```python
from build123d import *

# Parameters (mm, degrees)
SKETCH_1_W          = 38.4
SKETCH_1_H          = 30
EXTRUDE_1_DEPTH     = 2
CUT_EXTRUDE_1_DEPTH = 2
SKETCH_3_W          = 23
SKETCH_3_H          = 6
EXTRUDE_2_DEPTH     = 2
SKETCH_4_R          = 1.05
CUT_EXTRUDE_2_DEPTH = 2
SKETCH_5_W          = 7
SKETCH_5_H          = 3
EXTRUDE_3_DEPTH     = 2


with BuildPart() as part:
    # 草图1 → 凸台-拉伸1 (new body)
    with BuildSketch(Plane.XY):
        Rectangle(SKETCH_1_W, SKETCH_1_H)
    extrude(amount=EXTRUDE_1_DEPTH)

    # 草图2 → 切除-拉伸1 (cut)
    with BuildSketch(Plane(origin=(0, 0, 0), x_dir=(-1, 0, 0), z_dir=(0, 0, -1))):
        with BuildLine():
            Line((-12.2, 1.5), (-12.2, 15))
            Line((-12.2, 15), (12.2, 15))
            Line((12.2, 15), (12.2, 1.5))
            ThreePointArc((12.2, 1.5), (0, -10.7), (-12.2, 1.5))
        make_face()
    extrude(amount=-CUT_EXTRUDE_1_DEPTH, mode=Mode.SUBTRACT)

    # 草图3 → 凸台-拉伸2 (add)
    with BuildSketch(Plane(origin=(0, 0, 0), x_dir=(-1, 0, 0), z_dir=(0, 0, -1))):
        with Locations((0, -15)):
            Rectangle(SKETCH_3_W, SKETCH_3_H)
    extrude(amount=-EXTRUDE_2_DEPTH)

    # 草图4 → 切除-拉伸2 (cut)
    with BuildSketch(Plane.XY.offset(2)):
        with Locations((12.55, -15)):
            Circle(SKETCH_4_R)
        with Locations((-12.55, -15)):
            Circle(SKETCH_4_R)
    extrude(amount=-CUT_EXTRUDE_2_DEPTH, mode=Mode.SUBTRACT)

    # 草图5 → 凸台-拉伸3 (add)
    with BuildSketch(Plane(origin=(0, 0, 0), x_dir=(-1, 0, 0), z_dir=(0, 0, -1))):
        with Locations((-15.7, 16.5)):
            Rectangle(SKETCH_5_W, SKETCH_5_H)
        with Locations((15.7, 16.5)):
            Rectangle(SKETCH_5_W, SKETCH_5_H)
    extrude(amount=-EXTRUDE_3_DEPTH)


solid = part.part
```
For this review, take the finished solid that the model builds, in its own axes (mm). A direction names the side the tool comes from. Coordinates: 2 decimals unless noted, no trailing zeros. Write each loop counter-clockwise with the first axis right and the second up, starting at its lowest first coordinate (ties: lowest second). Pieces come first, ordered by that corner, then holes. Notation, with made-up numbers: (84, 20) - (100, 20) arc R24 cw to (100, 52) - close; hole circle Ø1 at (-19.75, 41.5). An arc over 180 degrees is marked (long way). Answer in a Markdown table with one row per item. Add a question column.
Q1. We need section B-B, the plane z = 0.6. State the section outline as (x, y) points.
Q2. We need section A-A, the plane y = 15.5. State the section outline as (x, z) points.
Q3. Tool access review of faces 1 (the flat face through (11.5, -17, 1)), 2 (the flat face through (-16, -15, 1)), 3 (the flat face through (12.2, 10, 1)): name each direction out of +Z, -Z, +X, -X, +Y, -Y from which nothing blocks a thin tool from reaching the whole face with its end or side.
Q4. We need section C-C, the plane y = -2.5. State the section outline as (x, z) points, and give its area (3 significant figures).
Q5. For P1, Ø1, axis at x = 15.5, z = 0.5, coming from the -Y side; P2, Ø0.6, axis at y = -16, z = 1, coming from the -X side, all flat-tipped, find the tip position at first contact; note any pin that passes through.
Q6. Draft analysis for pull direction X (two halves, no side actions). For faces 4 (the flat face through (0, -12, 0)), 5 (the flat face through (-19.2, 1, 1)), 6 (the cylindrical face through (12.57, -13.95, 1.01)), state which applies: +X half, -X half, draft (parallel to the pull), parting line (faces both ways), or undercut.
Q7. For probe 1 along X at (y, z) = (7, 0.7); probe 2 along X at (y, z) = (-4.5, 0.5); probe 3 along Y at (x, z) = (-16.5, 0.1), list the stretches that pass through material, from the lowest coordinate up.
Q8. We need section D-D, the plane x = 0. State the section outline as (y, z) points, and give its area (3 significant figures).
Answer list:
| question | item | result |
|---|---|---|
| 1 | outline | (-19.2, -15) - (-13.6, -15) arc R1.05 cw to (-11.5, -15) - (-11.5, -18) - (11.5, -18) - (11.5, -15) arc R1.05 cw to (13.6, -15) - (19.2, -15) - (19.2, 18) - (12.2, 18) - (12.2, 1.5) arc R12.2 cw to (-12.2, 1.5) - (-12.2, 18) - (-19.2, 18) - close |
| 2 | outline | (-19.2, 0) - (-12.2, 0) - (-12.2, 2) - (-19.2, 2) - close; (12.2, 0) - (19.2, 0) - (19.2, 2) - (12.2, 2) - close |
| 3 | face 1 | +Z, -Z, +X, -Y |
| 3 | face 2 | +Z, -Z, -X, -Y |
| 3 | face 3 | +Z, -Z, +Y |
| 4 | outline | (-19.2, 0) - (-11.53, 0) - (-11.53, 2) - (-19.2, 2) - close; (11.53, 0) - (19.2, 0) - (19.2, 2) - (11.53, 2) - close |
| 4 | area | 30.7 mm2 |
| 5 | P1 | stops at y = -15 |
| 5 | P2 | stops at x = -11.5 |
| 6 | face 4 | draft |
| 6 | face 5 | -X half |
| 6 | face 6 | undercut |
| 7 | probe 1 | x = -19.2 to -12.2, 12.2 to 19.2 |
| 7 | probe 2 | x = -19.2 to -10.62, 10.62 to 19.2 |
| 7 | probe 3 | y = -15 to 18 |
| 8 | outline | (-18, 0) - (-10.7, 0) - (-10.7, 2) - (-18, 2) - close |
| 8 | area | 14.6 mm2 |
